Model file for the job. Use its own axes, mm. A direction names the side the tool comes from. Coordinates: 2 decimals unless noted, no trailing zeros. Loops run counter-clockwise (first coordinate to the right, second up) from the corner with the lowest first, then second, coordinate; pieces in that order, holes last. Notation, with made-up numbers: M 75,42 L 108,42 A34 cw 108,72 Z; hole C 10,-40 d2. An arc over 180 degrees is marked long. One line per question, with ' | ' between items. Start each with the question number.
```python
from build123d import *

# Parameters (mm, degrees)
SKETCH1_W           = 8
SKETCH1_H           = 8
BOSS_EXTRUDE1_DEPTH = 8
SKETCH2_R           = 1.5
BOSS_EXTRUDE2_DEPTH = 3
SKETCH3_R           = 1.5
BOSS_EXTRUDE3_DEPTH = 3
SKETCH4_R           = 1.5
BOSS_EXTRUDE4_DEPTH = 3
SKETCH5_R           = 1.5
BOSS_EXTRUDE5_DEPTH = 3
FILLET3_R           = 1
FILLET4_R           = 1
FILLET5_R           = 1
FILLET6_R           = 1
FILLET7_R           = 1
FILLET8_R           = 1


with BuildPart() as part:
    # Sketch1 → Boss-Extrude1 (new body)
    with BuildSketch(Plane.XY):
        Rectangle(SKETCH1_W, SKETCH1_H)
    extrude(amount=BOSS_EXTRUDE1_DEPTH)

    # Sketch2 → Boss-Extrude2 (add)
    with BuildSketch(Plane(origin=(0, 4, 0), x_dir=(1, 0, 0), z_dir=(0, 1, 0))):
        with Locations((0, -4)):
            Circle(SKETCH2_R)
    extrude(amount=BOSS_EXTRUDE2_DEPTH)

    # Sketch3 → Boss-Extrude3 (add)
    with BuildSketch(Plane(origin=(4, 0, 0), x_dir=(0, 0, -1), z_dir=(1, 0, 0))):
        with Locations((-4, 0)):
            Circle(SKETCH3_R)
    extrude(amount=BOSS_EXTRUDE3_DEPTH)

    # Sketch4 → Boss-Extrude4 (add)
    with BuildSketch(Plane.XZ.offset(4)):
        with Locations((0, 4)):
            Circle(SKETCH4_R)
    extrude(amount=BOSS_EXTRUDE4_DEPTH)

    # Sketch5 → Boss-Extrude5 (add)
    with BuildSketch(Plane.ZY.offset(4)):
        with Locations((4, 0)):
            Circle(SKETCH5_R)
    extrude(amount=BOSS_EXTRUDE5_DEPTH)

    # Fillet3
    fillet3_edges = [part.edges().sort_by_distance(p)[0] for p in [
        (4, 0, 0),
    ]]
    fillet(fillet3_edges, radius=FILLET3_R)

    # Fillet4
    fillet4_edges = [part.edges().sort_by_distance(p)[0] for p in [
        (-4, 0, 0),
    ]]
    fillet(fillet4_edges, radius=FILLET4_R)

    # Fillet5
    fillet5_edges = [part.edges().sort_by_distance(p)[0] for p in [
        (-4, 0, 8),
    ]]
    fillet(fillet5_edges, radius=FILLET5_R)

    # Fillet6
    fillet6_edges = [part.edges().sort_by_distance(p)[0] for p in [
        (4, 0, 8),
    ]]
    fillet(fillet6_edges, radius=FILLET6_R)

    # Fillet7
    fillet7_edges = [part.edges().sort_by_distance(p)[0] for p in [
        (0, -4, 0),
        (-4, -4, 4),
        (0, -4, 8),
        (4, -4, 4),
    ]]
    fillet(fillet7_edges, radius=FILLET7_R)

    # Fillet8
    fillet8_edges = [part.edges().sort_by_distance(p)[0] for p in [
        (0, 4, 0),
        (-4, 4, 4),
        (0, 4, 8),
        (4, 4, 4),
    ]]
    fillet(fillet8_edges, radius=FILLET8_R)


solid = part.part
```
(1) Band-saw the part on B-B on z = 1.25. Write the cut outline in (x, y), then the cut area to 3 significant figures.
(2) Drill centre lines: line 1 (X direction, y = 3, z = 4); line 2 (Z direction, x = -0.25, y = 3.75). Where is each one in solid material? Low to high. Write a range as [from, to].
(3) 3-axis set-ups, long thin cutter, end or side, ignore diameter. For faces 1 (the face through (3.699, 0.042, 0.285)), 2 (the face through (4, -1.4, 2.6)), 3 (the face through (-4, -1.4, 2.6)): which of +Z, -Z, +X, -X, +Y, -Y reach the whole face in a straight line?
(4) Band-saw the part on D-D on y = -2.5. Write the cut outline in (x, z), then the cut area to 3 significant figures.
(5) Pin check, flat tips, straight feed: P1, Ø1.5, axis at x = -4.5, z = 3, coming from the -Y side; P2, Ø1.5, axis at y = 0, z = 7, coming from the +X side. Stop position of each tip, or through.
(6) Band-saw the part on A-A on y = 0. Write the cut outline in (x, z).
Computed values:
1) outline: M -4,-3 A1 ccw -3,-4 L 3,-4 A1 ccw 4,-3 L 4,3 A1 ccw 3,4 L -3,4 A1 ccw -4,3 Z | area: 63.1 mm^2
2) line 1: [-4, 4] | line 2: [0.34, 7.66]
3) face 1: -Z, +X, +Y, -Y | face 2: +X | face 3: -X
4) outline: M -4,1 A1 ccw -3,0 L 3,0 A1 ccw 4,1 L 4,7 A1 ccw 3,8 L -3,8 A1 ccw -4,7 Z | area: 63.1 mm^2
5) P1: y = -3.66 | P2: x = 4
6) outline: M -7,2.5 L -4,2.5 L -4,1 A1 ccw -3,0 L 3,0 A1 ccw 4,1 L 4,2.5 L 7,2.5 L 7,5.5 L 4,5.5 L 4,7 A1 ccw 3,8 L -3,8 A1 ccw -4,7 L -4,5.5 L -7,5.5 Z
